```python
from build123d import *

# Parameters (mm, degrees)
SKETCH1_R           = 3.937
BOSS_EXTRUDE1_DEPTH = 3.81


with BuildPart() as part:
    # Sketch1 → Boss-Extrude1 (new body, symmetric)
    with BuildSketch(Plane.XY):
        with BuildLine():
            Line((31.115, 6.858), (31.115, -22.352))
            Line((31.115, -22.352), (-31.115, -22.352))
            Line((-31.115, -22.352), (-31.115, -10.922))
            ThreePointArc((-31.115, -10.922), (-30.371051224, -9.125948776), (-28.575, -8.382))
            Line((-28.575, -8.382), (-25.049516684, -8.382))
            ThreePointArc((-25.049516684, -8.382), (-25.029149277, -8.382081661), (-25.008783181, -8.382326639))
            add(Edge.make_bspline(
                [(-25.008783181, -8.382326639), (-23.842012802, -8.401040323), (-18.102952542, -0.55711547), (-6.283660278, 15.246737848), (0.033942105, 22.061713275), (9.022065719, 22.599528271), (14.625326979, 21.304399973), (19.772057533, 10.818819135)],
                knots=[0.000772689, 0.000772689, 0.000772689, 0.000772689, 0.263254084, 0.33379531, 0.664808322, 0.734460983, 0.988945287, 0.988945287, 0.988945287, 0.988945287], degree=3))
            ThreePointArc((19.772057533, 10.818819135), (20.708902036, 9.782272814), (22.052196606, 9.398))
            Line((22.052196606, 9.398), (28.575, 9.398))
            ThreePointArc((28.575, 9.398), (30.371051224, 8.654051224), (31.115, 6.858))
        make_face()
        with Locations((5.334, 14.605)):
            Circle(SKETCH1_R, mode=Mode.SUBTRACT)
        with Locations((-24.892, -16.002)):
            Circle(SKETCH1_R, mode=Mode.SUBTRACT)
        with Locations((24.765, -16.002)):
            Circle(SKETCH1_R, mode=Mode.SUBTRACT)
    extrude(amount=BOSS_EXTRUDE1_DEPTH, both=True)


solid = part.part
```
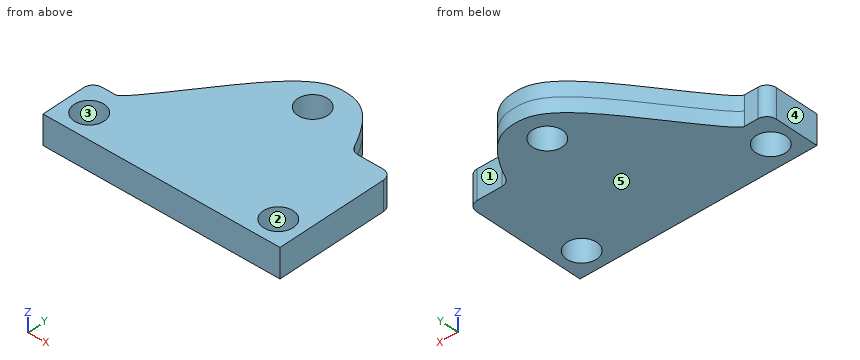
Could you check a few things on this model? Use its own coordinates, in mm. Face numbers are marked on the shaded views. A direction names the side the tool comes from. Coordinates: 2 decimals unless noted, no trailing zeros. Write each loop counter-clockwise with the first axis right and the second up, starting at its lowest first coordinate (ties: lowest second). Pieces come first, ordered by that corner, then holes. Notation, with made-up numbers: (27.25, -37) - (66.25, -37) arc R6 cw to (66.25, -27) - close; hole circle Ø1 at (-28.5, 53.5). An arc over 180 degrees is marked (long way). Use a Markdown table: item, result.
Q1. Imagine slicing it at B-B (z = -2). Count the separate pieces of the cut face and the enclosed holes in it, and give its area (3 significant figures).
Geometry check:
| item | result |
|---|---|
| separate pieces | 1 |
| enclosed holes | 3 |
| area | 1,860 mm2 |
Q2. Please list where these lines run through material, in increasing order: L1, parallel to X at y = -17.5, z = -2 (3 decimals); L2, parallel to X at y = -16.5, z = 2.5 (3 decimals); L3, parallel to Y at x = 6.5, z = 3.
Geometry check:
| item | result |
|---|---|
| L1 | x = -31.115 to -28.533, -21.251 to 21.124, 28.406 to 31.115 |
| L2 | x = -31.115 to -28.797, -20.987 to 20.86, 28.67 to 31.115 |
| L3 | y = -22.35 to 10.84, 18.37 to 22.38 |
Q3. Which directions (+Z, -Z, +X, -X, +Y, -Y) give clear straight access to the entire face, cutting with the end or side of a thin tool? Please do the marked faces 1 and 2.
Geometry check:
| item | result |
|---|---|
| face 1 | +Z, -Z, +X, +Y |
| face 2 | +Z, -Z |
Q4. I'm going to push flat-ended pins straight in: pin 1 Ø3 at (x, z) = (-8.5, 0) entering from +Y; pin 2 Ø1.8 at (x, z) = (-26, 1) entering from +Y; pin 3 Ø1.5 at (y, z) = (4.5, -1) entering from -X; pin 4 Ø7 at (x, y) = (-24.892, -16.002) entering from -Z (3 decimals). Where does each tip first touch, or does it pass through?
Geometry check:
| item | result |
|---|---|
| pin 1 | stops at y = 13.88 |
| pin 2 | stops at y = -8.38 |
| pin 3 | stops at x = -14.88 |
| pin 4 | passes through |
Q5. Thinking about a two-plate mould opening in X: for the marked faces 3, 4 and 5, which applies, +X half, -X half, draft (parallel to the pull), parting line (faces both ways), or undercut?
Geometry check:
| item | result |
|---|---|
| face 3 | undercut |
| face 4 | -X half |
| face 5 | draft |
Q6. Imagine slicing it at A-A (y = -17.5). List the corners of the cut face in (x, z) for me (3 decimals), and give its area (3 significant figures).
Geometry check:
| item | result |
|---|---|
| outline | (-31.115, -3.81) - (-28.533, -3.81) - (-28.533, 3.81) - (-31.115, 3.81) - close; (-21.251, -3.81) - (21.124, -3.81) - (21.124, 3.81) - (-21.251, 3.81) - close; (28.406, -3.81) - (31.115, -3.81) - (31.115, 3.81) - (28.406, 3.81) - close |
| area | 363 mm2 |
